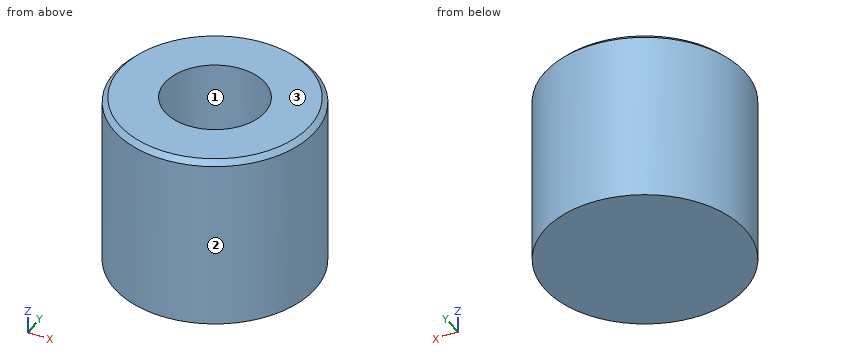
Autodesk Inventor part; units mm, degrees
ref_plane "YZ Plane" through (0, 0, 0) normal (1, 0, 0) x (0, 1, 0)
ref_plane "XZ Plane" through (0, 0, 0) normal (0, 1, 0) x (-1, 0, 0)
ref_plane "XY Plane" through (0, 0, 0) normal (0, 0, 1) x (1, 0, 0)
sketch "Sketch1" plane through (0, 0, 0) normal (0, 0, 1) x (1, 0, 0)
  circle A0 centre (0, 0) radius 20
  dimension "d0" = 40
extrude "Extrusion1" add sketch "Sketch1" along normal blind 35
sketch "Sketch5" plane through (0, 0, 35) normal (0, 0, 1) x (1, 0, 0)
  point P0 (0, 0)
  point P1 (0, 0)
hole "Hole2" at (0, 0, 35) direction (0, 0, -1) diameter 20 depth 22 tip angle 118
thread "Thread2"
chamfer "Chamfer1" distance 1 angle 45 1 edges at (-20, 0, 35)
properties part number "CompressionGrip"
Build history of the part. All positions in model axes, mm. Face numbers are marked on the shaded views. Give positions to 0.01 mm unless a question says otherwise; leave off trailing zeros. Order: outer loops, then holes, each group sorted by start corner. A loop starts at its lowest first (then second) coordinate and runs counter-clockwise, first axis right, second up. Notation, with made-up numbers: M -25,52.25 L 31,52.25 A6 cw 31,58.25 Z; hole C -10.75,7 d7. An arc over 180 degrees is marked long. Use one line per item in the form item = value.
Q1. Slice it at A-A, the plane z = 18.5. Write the cut outline in (x, y).
Conclusion:
outline = C 0,0 d40; hole C 0,0 d20
Q2. Pin check, flat tips, straight feed: P1, Ø6, axis at x = 2, z = 22.5, coming from the -Y side; P2, Ø2, axis at y = -5.5, z = 19.5, coming from the +X side; P3, Ø12, axis at x = 8.5, z = 17, coming from the -Y side. Stop position of each tip, or through.
Conclusion:
P1 = -20
P2 = 19.49
P3 = -19.84
Q3. Slice it at B-B, the plane z = 4. Write the cut outline in (x, y), and give its area (3 significant figures).
Conclusion:
outline = C 0,0 d40
area = 1,260 mm2
Q4. Pull direction Y, two halves, no side cores. Call the marked faces 1, 2 and 3: released by +Y, released by -Y, zero draft, split by the parting line, or undercut.
Conclusion:
face_1 = undercut
face_2 = split by the parting line
face_3 = zero draft
Q5. Wall check: probe 1 along Y at (x, z) = (0, 24); probe 2 along Y at (x, z) = (9, 32.5); probe 3 along X at (y, z) = (-3, 18). Give the ranges that are in metal, low to high.
Conclusion:
probe_1 = -20 to -10, 10 to 20
probe_2 = -17.86 to -4.36, 4.36 to 17.86
probe_3 = -19.77 to -9.54, 9.54 to 19.77
